Geometry: final body of the model. Coordinates: model frame, mm. A direction names the side the tool comes from. Give positions to 0.01 mm unless a question says otherwise; leave off trailing zeros. Order: outer loops, then holes, each group sorted by start corner. A loop starts at its lowest first (then second) coordinate and runs counter-clockwise, first axis right, second up. Notation, with made-up numbers: M 85.5,60.5 L 143.5,60.5 A16 cw 143.5,85.5 Z; hole C -32.5,21.5 d5. An arc over 180 degrees is marked long. Use CSV: the item, a comma, the result in double quotes.
Solid Edge part; units mm, degrees
sketch "Sketch1" plane through (0, 0, 0) normal (0, -1, 0) x (1, 0, 0)
  line L0 (21, 16.97) -> (16.97, 21)
  line L1 (16.97, 21) -> (-16.97, 21)
  line L2 (-16.97, 21) -> (-21, 16.97)
  line L3 (-21, 16.97) -> (-21, -16.97)
  line L4 (-21, -16.97) -> (-16.97, -21)
  line L5 (-16.97, -21) -> (16.97, -21)
  line L6 (16.97, -21) -> (21, -16.97)
  line L7 (21, -16.97) -> (21, 16.97)
  line L8 (26, 19.0411) -> (19.0411, 26)
  line L9 (19.0411, 26) -> (-19.0411, 26)
  line L10 (-19.0411, 26) -> (-26, 19.0411)
  line L11 (-26, 19.0411) -> (-26, -19.0411)
  line L12 (-26, -19.0411) -> (-19.0411, -26)
  line L13 (-19.0411, -26) -> (19.0411, -26)
  line L14 (19.0411, -26) -> (26, -19.0411)
  line L15 (26, -19.0411) -> (26, 19.0411)
extrude "Protrusion1" add sketch "Sketch1" against normal blind 35
sketch "Sketch2" plane through (0, 0, 0) normal (0, -1, 0) x (1, 0, 0)
  line L0 (19.0411, 26) -> (-19.0411, 26)
  line L1 (-19.0411, 26) -> (-26, 19.0411)
  line L2 (-26, 19.0411) -> (-26, -19.0411)
  line L3 (-26, -19.0411) -> (-19.0411, -26)
  line L4 (-19.0411, -26) -> (19.0411, -26)
  line L5 (19.0411, -26) -> (26, -19.0411)
  line L6 (26, -19.0411) -> (26, 19.0411)
  line L7 (26, 19.0411) -> (19.0411, 26)
extrude "Deckel" add sketch "Sketch2" along normal blind 5
hole "Motorwelle" at (0, -5, 0) direction (0, 1, 0) diameter 6 end up to next
hole "Hole1" at (-15.5, -5, -15.5) direction (0, 1, 0) diameter 3.2 end up to next start chamfer 0.2 start chamfer angle 45
hole "Hole2" at (-15.5, -5, 15.5) direction (0, 1, 0) diameter 3.2 end up to next start chamfer 0.2 start chamfer angle 45
hole "Hole3" at (15.5, -5, 15.5) direction (0, 1, 0) diameter 3.2 end up to next start chamfer 0.2 start chamfer angle 45
hole "Hole4" at (15.5, -5, -15.5) direction (0, 1, 0) diameter 3.2 end up to next start chamfer 0.2 start chamfer angle 45
sketch "Sketch3" plane through (0, 0, 0) normal (0, 1, 0) x (0, 0, 1)
  circle A0 centre (0, 0) radius 11.5
extrude "Motoflansch" cut sketch "Sketch3" against normal blind 1
sketch "Sketch4" plane through (0, -5, 0) normal (0, -1, 0) x (1, 0, 0)
  line L0 (-26, 19.0411) -> (-19.0411, 26)
  line L1 (-19.0411, 26) -> (4, 26)
  line L2 (4, 26) -> (4, 56)
  line L3 (-26, 56) -> (4, 56)
  line L4 (-26, 19.0411) -> (-26, 56)
  dimension "D1" = 4
  dimension "D2" = 26
extrude "Motoraufhängung_Leiste" add sketch "Sketch4" against normal blind 23
sketch "Sketch5" plane through (-13, 18, 33.5205) normal (0, 1, 0) x (-1, 0, 0)
  line L0 (-17, -7.5205) -> (-17, 22.4795)
  line L1 (-17, 22.4795) -> (-12, 22.4795)
  line L2 (-12, 22.4795) -> (-12, -7.5205)
  line L3 (-12, -7.5205) -> (-17, -7.5205)
  dimension "D1" = 17
extrude "Zentrierung_Leiste" add sketch "Sketch5" along normal blind 17.5
sketch "Sketch6" plane through (0, -5, 11) normal (0, -1, 0) x (1, 0, 0)
  line L0 (-26, -30.0411) -> (-26, 8.0411)
  line L1 (-26, 8.0411) -> (-63, 8.0411)
  line L2 (-66, 5.0411) -> (-63, 8.0411)
  line L3 (-66, 5.0411) -> (-66, -27.0411)
  line L4 (-63, -30.0411) -> (-66, -27.0411)
  line L5 (-63, -30.0411) -> (-26, -30.0411)
  dimension "D1" = 63
  dimension "D2" = 66
  dimension "D3" = 66
extrude "Auflage_auf_Platte" add sketch "Sketch6" against normal blind 23
hole "Bohrung_Alustange" at (-11, 5, 56) direction (0, 0, -1) diameter 8 depth 11 tip angle 118 start chamfer 0.2 start chamfer angle 45
sketch "Sketch7" plane through (0, 35, 0) normal (0, 1, 0) x (1, 0, 0)
  line L0 (-19.0411, 26) -> (-16.97, 21)
  line L1 (-16.97, 21) -> (-16.97, -21)
  line L2 (-16.97, -21) -> (-19.0411, -26)
  line L3 (-19.0411, -26) -> (-26, -26)
  line L4 (-26, -26) -> (-26, 26)
  line L5 (-26, 26) -> (-19.0411, 26)
extrude "Motorseite" cut sketch "Sketch7" against normal blind 17
hole "Hole5" at (-8, -5, 32) direction (0, 1, 0) diameter 4.3 end up to next
hole "Hole6" at (-15, -5, 41) direction (0, 1, 0) diameter 4.3 end up to next
hole "Hole7" at (-59, -5, 12.0411) direction (0, 1, 0) diameter 4.3 end up to next
hole "Hole8" at (-59, -5, -12.0411) direction (0, 1, 0) diameter 4.3 end up to next
hole "Hole9" at (-46, -5, 0) direction (0, 1, 0) diameter 4.3 end up to next
fillet "Verrundung_Innen" radius 3 3 edges at (-26, 6.5, -19.0411) (-26, 6.5, 19.0411) (4, 15, 26)
fillet "Verrundung_spitzeEcke" radius 5 2 edges at (-19.0411, 26.5, 26) (-19.0411, 26.5, -26)
1. Section A-A, the plane x = -46. Return the cut outline in (y, z), plus the area to 3 significant figures.
Answer:
outline,"M -5,-19.04 L 18,-19.04 L 18,-2.15 L -5,-2.15 Z; M -5,2.15 L 18,2.15 L 18,19.04 L -5,19.04 Z"
area,"777 mm2"
2. Line query: line 1 (Z direction, x = -59, y = 12); line 2 (X direction, y = -3.4, z = -15.5); line 3 (Z direction, x = 15.5, y = -2). Output: solid intervals per line, ascending.
Answer:
line 1,"-19.04 to -14.19, -9.89 to 9.89, 14.19 to 19.04"
line 2,"-66 to -17.1, -13.9 to 13.9, 17.1 to 26"
line 3,"-26 to -17.1, -13.9 to 13.9, 17.1 to 26"
3. Section C-C, the plane z = 41. Return the cut outline in (x, y).
Answer:
outline,"M -26,-5 L -17.15,-5 L -17.15,18 L -26,18 Z; M -12.85,-5 L 4,-5 L 4,35.5 L -1,35.5 L -1,18 L -12.85,18 Z"
4. Reachability of faces 1 (the face through (-6, 26, 26)), 2 (the face through (16.58, -2.43, 16.68)), 3 (the face through (-2.4, -1, 2.4)), 4 (the face through (-26, 6, 39)) from +Z, -Z, +X, -X, +Y, -Y: full face, straight path, thin tool, end or side. Return the list, or none.
Answer:
face 1,"+Z, -X, +Y"
face 2,"+Y, -Y"
face 3,"+Y"
face 4,"+Z, -X, +Y, -Y"
5. Pin query (flat end, axial travel): pin 1 Ø4 at (x, z) = (-15.5, -15.5) entering from +Y; pin 2 Ø5 at (x, z) = (-7, 4) entering from +Y; pin 3 Ø19 at (y, z) = (28.5, 45.5) entering from -X. Return the tip coordinate at first contact, or that it passes through.
Answer:
pin 1,"y = 0"
pin 2,"y = -1"
pin 3,"x = -1"
6. Pull-direction query (X, two-part tool) for faces 5 (the face through (-14.42, -2.43, 16.68)), 6 (the face through (2, 35.5, 41)), 7 (the face through (-19.01, 8.87, -18.96)), 8 (the face through (-26.079, 6.339, -19.276)); classes: +X half, -X half, draft (parallel to the pull), parting line (faces both ways), or undercut.
Answer:
face 5,"undercut"
face 6,"draft"
face 7,"undercut"
face 8,"-X half"
7. Section B-B, the plane z = 0. Return the cut outline in (x, y), plus the area to 3 significant figures.
Answer:
outline,"M -66,-5 L -48.15,-5 L -48.15,18 L -66,18 Z; M -43.85,-5 L -3,-5 L -3,-1 L -11.5,-1 L -11.5,0 L -21,0 L -21,18 L -43.85,18 Z; M 3,-5 L 26,-5 L 26,35 L 21,35 L 21,0 L 11.5,0 L 11.5,-1 L 3,-1 Z"
area,"1,300 mm2"
8. Section D-D, the plane z = 50.5. Return the cut outline in (x, y), plus the area to 3 significant figures.
Answer:
outline,"M -26,-5 L 4,-5 L 4,35.5 L -1,35.5 L -1,18 L -26,18 Z; hole C -11,5 d8"
area,"727 mm2"
